```python
from build123d import *

# Parameters (mm, degrees)
SKETCH2_W          = 0.381
SKETCH2_H          = 3.9624
SKETCH4_W          = 61.9252
SKETCH4_H          = 30.9626
SKETCH4_W_2        = 30.9626
SKETCH4_H_2        = 12.573
CUT_EXTRUDE1_DEPTH = 4.6482


with BuildPart() as part:
    # Sketch1 → Revolve1 (revolve)
    with BuildSketch(Plane.XY):
        Polygon((0, 0), (0, 6.50875), (0.762, 7.27075), (2.7178, 7.27075), (3.3528, 6.63575), (3.9878, 6.63575), (3.9878, 7.74065), (11.938, 7.74065), (12.7, 6.97865), (12.7, 0), align=None)
    revolve(axis=Axis((12.7, 0, 0), (-1, 0, 0)))

    # Sketch2 → Cut-Revolve1 (revolve, cut)
    with BuildSketch(Plane.XY):
        with Locations((12.5095, 1.9812)):
            Rectangle(SKETCH2_W, SKETCH2_H)
    revolve(axis=Axis((12.7, 0, 0), (-1, 0, 0)), mode=Mode.SUBTRACT)

    # Sketch3 → Cut-Revolve2 (revolve, cut)
    with BuildSketch(Plane.XY):
        Polygon((0, 0), (0, 1.98374), (11.88974, 1.98374), (12.319, 2.413), (12.319, 0), align=None)
    revolve(axis=Axis((12.319, 0, 0), (-1, 0, 0)), mode=Mode.SUBTRACT)

    # Sketch4 → Cut-Extrude1 (cut)
    with BuildSketch(Plane(origin=(12.7, 0, 0), x_dir=(0, 0, -1), z_dir=(1, 0, 0))):
        Rectangle(SKETCH4_W, SKETCH4_H)
        Rectangle(SKETCH4_W_2, SKETCH4_H_2, mode=Mode.SUBTRACT)
    extrude(amount=-CUT_EXTRUDE1_DEPTH, mode=Mode.SUBTRACT)

    # Sketch5 → Revolve2 (revolve)
    with BuildSketch(Plane.XY):
        with BuildLine():
            Line((3.230093808, 7.74065), (3.230093808, 7.656481804))
            Line((3.230093808, 7.656481804), (3.870760245, 7.015815367))
            ThreePointArc((3.870760245, 7.015815367), (3.907957684, 6.926012806), (3.870760245, 6.836210245))
            Line((3.870760245, 6.836210245), (3.6703, 6.63575))
            Line((3.6703, 6.63575), (3.3528, 6.63575))
            Line((3.3528, 6.63575), (3.3528, 6.38175))
            Line((3.3528, 6.38175), (3.9878, 6.38175))
            Line((3.9878, 6.38175), (3.9878, 7.186143808))
            Line((3.9878, 7.186143808), (3.433293808, 7.74065))
            Line((3.433293808, 7.74065), (3.230093808, 7.74065))
        make_face()
    revolve(axis=Axis((3.9878, 0, 0), (-1, 0, 0)))


solid = part.part
```
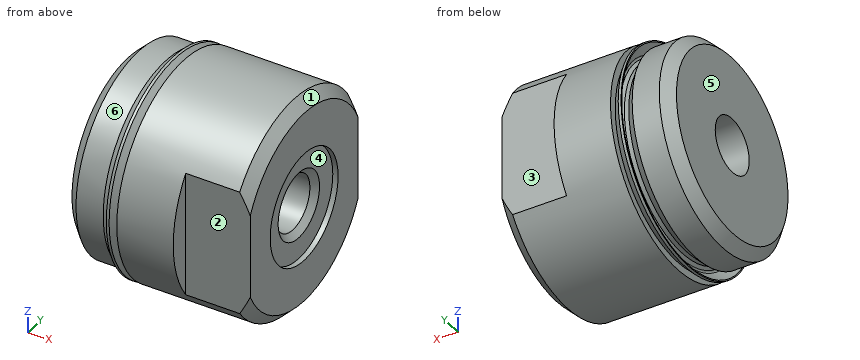
Here's how the part is built. I have some questions about the finished solid (model axes, mm). Face numbers are marked on the shaded views. A direction names the side the tool comes from. Coordinates: 2 decimals unless noted, no trailing zeros. Loops run counter-clockwise (first coordinate to the right, second up) from the corner with the lowest first, then second, coordinate; pieces in that order, holes last. Notation, with made-up numbers: (34.25, 64) - (72.25, 64) arc R17 cw to (72.25, 68) - close; hole circle Ø11 at (76.25, 60.5). An arc over 180 degrees is marked (long way). Answer as CSV lines item,"result".
Q1. If we section it at B-B, the plane x = 5.25: Write out the boundary of the cut face in (y, z), and give its area (3 significant figures).
Response:
outline,"circle Ø15.48 at (0, 0); hole circle Ø3.97 at (0, 0)"
area,"176 mm2"
Q2. We'd pull the mould along Z, two halves only. Please class the marked faces 4, 5 and 6: pulls with the +Z half, pulls with the -Z half, needs draft (parallel to the pull), parting line crosses it, or undercut.
Response:
face 4,"undercut"
face 5,"needs draft"
face 6,"parting line crosses it"
Q3. If I drill on L1, parallel to Y at x = 12.6, z = 0; L2, parallel to Z at x = 3.5, y = -6; L3, parallel to Y at x = 5.5, z = 0, over which ranges is the centre line in solid material (lowest first)? Write a range as [from, to].
Response:
L1,"[-6.29, -3.96], [3.96, 6.29]"
L2,"[-4.78, -4.31], [-2.83, 2.83], [4.31, 4.78]"
L3,"[-7.74, -1.98], [1.98, 7.74]"
Q4. For the marked faces 1, 2 and 3, which set-ups out of +Z, -Z, +X, -X, +Y, -Y let a thin tool reach every point of the face, with its end or its side?
Response:
face 1,"+Z, +X"
face 2,"+Z, -Z, +X, -Y"
face 3,"+Z, -Z, +X, +Y"
Q5. For pin 1 (1 mm diameter, centred on x = 6.5, y = -5, fed in from -Z); pin 2 (1.2 mm diameter, centred on y = -7, z = 0, fed in from +X); pin 3 (2.5 mm diameter, centred on x = 10.5, z = -2, fed in from +Y), each with a flat end and sliding along its axis, tell me the tip position at first contact or that it passes through.
Response:
pin 1,"z = -6.3"
pin 2,"x = 8.05"
pin 3,"y = 6.29"
Q6. If we section it at A-A, the plane x = 10.25: Write out the boundary of the cut face in (y, z), and give its area (3 significant figures).
Response:
outline,"(-6.29, -4.52) arc R7.74 ccw to (6.29, -4.52) - (6.29, 4.52) arc R7.74 ccw to (-6.29, 4.52) - close; hole circle Ø3.97 at (0, 0)"
area,"158 mm2"
